Part model, mm, in its own coordinate system. A direction names the side the tool comes from. Give positions to 0.01 mm unless a question says otherwise; leave off trailing zeros. Write each loop counter-clockwise with the first axis right and the second up, starting at its lowest first coordinate (ties: lowest second). Pieces come first, ordered by that corner, then holes. Notation, with made-up numbers: M 39,-5 L 94,-5 A14 ccw 94,19 Z; hole C 87.5,53.25 d6. An arc over 180 degrees is marked long. Use CSV: the item, a comma, the result in double quotes. Start each with the question number.
1. Band-saw the part on D-D, the plane x = 2.5. List the corners of the cut face in (y, z).
2. Mould opens along X. For faces 1 (the face through (76.958, 8.25, -25.715)), 2 (the face through (-2, 23, -23)), 3 (the face through (-3.968, 16.518, -101.656)) say: pulls with the +X half, pulls with the -X half, needs draft (parallel to the pull), parting line crosses it, or undercut.
3. Drill centre lines: line 1 along Y through (x, z) = (-6, -7); line 2 along Y through (x, z) = (-3, -102); line 3 along Z through (x, y) = (76.9, 23). Where is each one in solid material? Low to high. Write a range as from..to.
4. Band-saw the part on B-B, the plane z = -15. List the corners of the cut face in (x, y), then the cut area to 3 significant figures.
5. 3-axis set-ups, long thin cutter, end or side, ignore diameter. For faces 4 (the face through (69.436, 27.075, -37.656)), 5 (the face through (-2, 15, -15)), 6 (the face through (74, 8, -28)): which of +Z, -Z, +X, -X, +Y, -Y reach the whole face in a straight line?
6. Band-saw the part on A-A, the plane x = 29.66. List the corners of the cut face in (y, z), then the cut area to 3 significant figures.
7. Band-saw the part on C-C, the plane z = -52. List the corners of the cut face in (x, y), then the cut area to 3 significant figures.
8. Drop flat-ended pins along their axis: pin 1 Ø3 at (y, z) = (23, -23) entering from -X; pin 2 Ø12 at (y, z) = (8.5, -67.5) entering from +X; pin 3 Ø2.5 at (x, y) = (67.75, 10) entering from -Z. Give the stop position or say it passes through.
from build123d import *

# Parameters (mm, degrees)
SKETCH_1_W          = 72
SKETCH_1_H          = 30
EXTRUDE_1_DEPTH     = 8
SKETCH_2_W          = 113.6
SKETCH_2_H          = 30
EXTRUDE_2_DEPTH     = 8
SKETCH_3_W          = 49.6
SKETCH_3_H          = 30
EXTRUDE_3_DEPTH     = 8
SKETCH_5_W          = 18.5
SKETCH_5_H          = 30
SKETCH_5_R          = 2
EXTRUDE_4_DEPTH     = 8
SKETCH_10_R         = 2
CUT_EXTRUDE_3_DEPTH = 15.5
SKETCH_11_R         = 2
CUT_EXTRUDE_4_DEPTH = 6
SKETCH_12_R         = 1.8
CUT_EXTRUDE_6_DEPTH = 8
CUT_EXTRUDE_START   = -6
SKETCH_13_R         = 2
CUT_EXTRUDE_7_DEPTH = 6


with BuildPart() as part:
    # 草圖1 → 填料-伸長1 (new body)
    with BuildSketch(Plane.XY):
        with Locations((36, 15)):
            Rectangle(SKETCH_1_W, SKETCH_1_H)
    extrude(amount=EXTRUDE_1_DEPTH)

    # 草圖2 → 填料-伸長2 (add)
    with BuildSketch(Plane.ZY):
        with Locations((-48.8, 15)):
            Rectangle(SKETCH_2_W, SKETCH_2_H)
    extrude(amount=EXTRUDE_2_DEPTH)

    # 草圖3 → 填料-伸長3 (add)
    with BuildSketch(Plane(origin=(72, 0, 0), x_dir=(0, 0, -1), z_dir=(1, 0, 0))):
        with Locations((16.8, 15)):
            Rectangle(SKETCH_3_W, SKETCH_3_H)
    extrude(amount=EXTRUDE_3_DEPTH)

    # 草圖5 → 填料-伸長4 (add)
    with BuildSketch(Plane(origin=(0, 0, -41.6), x_dir=(-1, 0, 0), z_dir=(0, 0, -1))):
        with Locations((-70.75, 15)):
            Rectangle(SKETCH_5_W, SKETCH_5_H)
        with Locations(Location((-67.75, 26, 0), (0, 0, 90))):
            Circle(SKETCH_5_R, mode=Mode.SUBTRACT)
        with Locations(Location((-67.75, 18, 0), (0, 0, 90))):
            Circle(SKETCH_5_R, mode=Mode.SUBTRACT)
        with Locations(Location((-67.75, 10, 0), (0, 0, 90))):
            Circle(SKETCH_5_R, mode=Mode.SUBTRACT)
    extrude(amount=-EXTRUDE_4_DEPTH)

    # 草圖10 → 除料-伸長3 (cut)
    with BuildSketch(Plane.XY.offset(8)):
        with Locations((29.66, 23)):
            Circle(SKETCH_10_R)
        with Locations((37.66, 23)):
            Circle(SKETCH_10_R)
        with Locations((37.66, 7)):
            Circle(SKETCH_10_R)
        with Locations((29.66, 7)):
            Circle(SKETCH_10_R)
    extrude(amount=-CUT_EXTRUDE_3_DEPTH, mode=Mode.SUBTRACT)

    # 草圖11 → 除料-伸長4 (cut)
    with BuildSketch(Plane.ZY.offset(8)):
        with Locations((-31, 23)):
            Circle(SKETCH_11_R)
        with Locations((-31, 15)):
            Circle(SKETCH_11_R)
        with Locations((-31, 7)):
            Circle(SKETCH_11_R)
        with Locations((-23, 23)):
            Circle(SKETCH_11_R)
        with Locations((-23, 15)):
            Circle(SKETCH_11_R)
        with Locations((-23, 7)):
            Circle(SKETCH_11_R)
        with Locations((-15, 23)):
            Circle(SKETCH_11_R)
        with Locations((-15, 15)):
            Circle(SKETCH_11_R)
        with Locations((-15, 7)):
            Circle(SKETCH_11_R)
        with Locations((-7, 23)):
            Circle(SKETCH_11_R)
        with Locations((-7, 15)):
            Circle(SKETCH_11_R)
        with Locations((-7, 7)):
            Circle(SKETCH_11_R)
    extrude(amount=-CUT_EXTRUDE_4_DEPTH, mode=Mode.SUBTRACT)

    # 草圖12 → 除料-伸長6 (cut)
    with BuildSketch(Plane(origin=(0, 0, -105.6), x_dir=(-1, 0, 0), z_dir=(0, 0, -1))):
        with Locations((3, 23)):
            Circle(SKETCH_12_R)
        with Locations((3, 15)):
            Circle(SKETCH_12_R)
        with Locations((3, 7)):
            Circle(SKETCH_12_R)
    extrude(amount=-CUT_EXTRUDE_6_DEPTH, mode=Mode.SUBTRACT)

    # 草圖13 → 除料-伸長7 (cut)
    with BuildSketch(Plane(origin=(80, 0, 0), x_dir=(0, 0, -1), z_dir=(1, 0, 0)).offset(CUT_EXTRUDE_START)):
        with Locations(Location((7, 23, 0), (0, 0, 180))):
            Circle(SKETCH_13_R)
        with Locations((11.115966043, 16.140056594)):
            Circle(SKETCH_13_R)
        with Locations((11.713009493, 8.162366508)):
            Circle(SKETCH_13_R)
        with Locations(Location((15, 23, 0), (0, 0, 180))):
            Circle(SKETCH_13_R)
        with Locations((19.115966043, 16.140056594)):
            Circle(SKETCH_13_R)
        with Locations((19.713009493, 8.162366508)):
            Circle(SKETCH_13_R)
        with Locations(Location((23, 23, 0), (0, 0, 180))):
            Circle(SKETCH_13_R)
        with Locations((27.115966043, 16.140056594)):
            Circle(SKETCH_13_R)
        with Locations((27.713009493, 8.162366508)):
            Circle(SKETCH_13_R)
        with Locations(Location((31, 23, 0), (0, 0, 180))):
            Circle(SKETCH_13_R)
        with Locations((35.115966043, 16.140056594)):
            Circle(SKETCH_13_R)
        with Locations((35.713009493, 8.162366508)):
            Circle(SKETCH_13_R)
    extrude(amount=CUT_EXTRUDE_7_DEPTH, mode=Mode.SUBTRACT)


solid = part.part
Output:
1,outline,"M 0,0 L 30,0 L 30,8 L 0,8 Z"
2,face 1,"needs draft"
2,face 2,"pulls with the -X half"
2,face 3,"undercut"
3,line 1,"y = 0..5, 9..13, 17..21, 25..30"
3,line 2,"y = 0..5.2, 8.8..13.2, 16.8..21.2, 24.8..30"
3,line 3,"z = -41.6..-33, -29..-25, -21..-17, -13..-9, -5..8"
4,outline,"M -8,0 L 0,0 L 0,30 L -8,30 L -8,25 L -2,25 L -2,21 L -8,21 L -8,17 L -2,17 L -2,13 L -8,13 L -8,9 L -2,9 L -2,5 L -8,5 Z; M 72,0 L 80,0 L 80,21 L 74,21 L 74,25 L 80,25 L 80,30 L 72,30 Z"
4,area,"384 mm²"
5,face 4,"-Z"
5,face 5,"-X"
5,face 6,"+X"
6,outline,"M 0,0 L 5,0 L 5,8 L 0,8 Z; M 9,0 L 21,0 L 21,8 L 9,8 Z; M 25,0 L 30,0 L 30,8 L 25,8 Z"
6,area,"176 mm²"
7,outline,"M -8,0 L 0,0 L 0,30 L -8,30 Z"
7,area,"240 mm²"
8,pin 1,"stops at x = -2"
8,pin 2,"stops at x = 0"
8,pin 3,"stops at z = 0"
